Autodesk Inventor part; units mm, degrees
ref_plane "Work Plane2" through (0, 0, 0) normal (-1, 0, 0) x (0, 1, 0)
ref_plane "Work Plane3" through (0, 3.5, 0) normal (0, 1, 0) x (1, 0, 0)
ref_plane "YZ Plane" through (0, 0, 0) normal (1, 0, 0) x (0, 1, 0)
sketch "Sketch3" plane through (0, 0, 0) normal (1, 0, 0) x (0, 1, 0)
  line L0 (0, 0) -> (0, -11) construction
  line L1 (0, 0) -> (7, 0) construction
  line L2 (7, 0) -> (7, -11) construction
  line L3 (0, -11) -> (0, -41.91)
  line L4 (0, -41.91) -> (-1.9706, -41.91) construction
  line L5 (0, -11) -> (7, -11)
  line L6 (7, -11) -> (7, -41.91)
  line L7 (0, -41.91) -> (0, -39.6842) construction
  line L8 (0, -41.91) -> (7, -41.91)
  dimension "d7" = 7
  dimension "d8" = 11
  dimension "d9" = 41.91
revolve "Revolution1" add sketch "Sketch3" angle 360 about axis through (0, 0, 0) along (0, 1, 0)
ref_plane "Work Plane2" through (0, 0, 0) normal (-1, 0, 0) x (0, 1, 0)
sketch "Sketch4" plane through (0, 0, 0) normal (-1, 0, 0) x (0, 1, 0)
  line L0 (0, 0) -> (7, 0)
  line L1 (7, 41.91) -> (7, -41.91)
  line L2 (7, 0) -> (7, 11)
  line L3 (7, 0) -> (8, 0)
  line L4 (8, 0) -> (8, 15)
  line L5 (8, 15) -> (7, 15)
  line L6 (8, 15) -> (8, 41.91)
  line L7 (8, 41.91) -> (7, 41.91)
  line L8 (0, 0) -> (0, 0.75)
  line L9 (0, 11) -> (0, -11)
  line L10 (8, 15) -> (0, 15)
  line L11 (0, 41.91) -> (0, -41.91)
  line L12 (0, 15) -> (-1, 15)
  line L13 (-1, 15) -> (-1, 41.91)
  line L14 (-1, 41.91) -> (0, 41.91)
  dimension "d16" = 11
  dimension "d17" = 1
  dimension "d18" = 15
  dimension "d20" = 0.75
  dimension "d21" = 1
ref_plane "Work Plane3" through (0, 3.5, 0) normal (0, 1, 0) x (1, 0, 0)
revolve "Revolution2" add sketch "Sketch4" angle 360 about axis through (0, 0, 0) along (0, 1, 0) contours L12 L13 L14 L11 | L1 L7 L6 L5
sketch "Sketch5" plane through (0, 8, 0) normal (0, 1, 0) x (1, 0, 0)
  circle A0 centre (0, 0) radius 18.175
  circle A1 centre (0, 0) radius 15
  circle A2 centre (0, 0) radius 41.91
  circle A3 centre (0, 0) radius 35.56
  dimension "d22" = 3.175
  dimension "d23" = 6.35
extrude "Extrusion2" cut sketch "Sketch5" against normal through all contours A3
sketch "Sketch6" plane through (0, 8, 0) normal (0, 1, 0) x (1, 0, 0)
  circle A0 centre (0, 0) radius 18.175
  circle A1 centre (0, 0) radius 35.56
  line L0 (16.0245, 8.5759) -> (30.4464, -18.372)
  line L1 (27.5834, -22.4426) -> (17.7246, -4.0211)
  dimension "d26" = 4.445
extrude "Extrusion3" add sketch "Sketch6" against normal up to surface (9 mm away) contours A0 L0 A1 L1 picked at (22.1844, -5.1361)
pattern_circular "Circular Pattern1" count 3 over 360 about axis through (0, 3.5, 0) along (0, -1, 0) of "Extrusion3"
fillet "Fillet1" radius 6.35 3 edges at (-5.3799, 3.5, -17.3605) (17.7246, 3.5, 4.0211) (-12.3447, 3.5, 13.3394)
fillet "Fillet1" radius 3.175 3 edges at (27.5834, 3.5, 22.4426) (-33.2276, 3.5, 12.6666) (5.6442, 3.5, -35.1092)
fillet "Fillet1" radius 3.175 3 edges at (0.6874, 3.5, -35.5534) (-31.1338, 3.5, 17.1814) (30.4464, 3.5, 18.372)
sketch "Sketch7" plane through (0, 0, 0) normal (-1, 0, 0) x (0, 1, 0)
  line L0 (8, -41.91) -> (8, 41.91)
  line L1 (-1, -41.91) -> (-1, 41.91)
  line L2 (8, -41.91) -> (-1, -41.91)
  arc A0 (6.04, -41.91) -> (8, -35.56) centre (-3.2664, -35.56) ccw
  arc A1 (-1, -35.56) -> (0.96, -41.91) centre (10.2664, -35.56) ccw
  line L3 (0.96, -41.91) -> (6.04, -41.91)
  line L4 (-1, -35.56) -> (8, -35.56)
  line L5 (8, -22.57) -> (-1, -22.57)
  line L6 (8, -24.1718) -> (8, -35.56)
  line L7 (-1, -24.1718) -> (8, -24.1718)
  line L8 (-1, -22.57) -> (-1, -24.1718)
  line L9 (8, -35.56) -> (8, -35.56)
  line L10 (0, 0) -> (11.7377, 0)
  dimension "d36" = 6.35
  dimension "d37" = 5.08
revolve "Revolution3" cut sketch "Sketch7" angle 360 about axis through (0, 0, 0) along (0, 1, 0) contours L2 A0 L0 | A1 L2 L1
fillet "Fillet2" radius 1.5875 4 edges at (41.91, 6.04, 0) (-41.91, 6.04, 0) (-41.91, 0.96, 0) (41.91, 0.96, 0)
sketch "Sketch8" plane through (27.5145, 8, 12.8937) normal (0, 1, 0) x (0.8816766, 0, -0.4718541)
  circle A0 centre (-18.175, 24.3509) radius 19.05
  arc A1 (-27.2625, 8.6109) -> (-12.7058, 7.0183) centre (-18.175, 24.3509) ccw
  dimension "d40" = 38.1
sketch "Sketch9" plane through (27.5145, 8, 12.8937) normal (0, 1, 0) x (0.8816766, 0, -0.4718541)
  circle A0 centre (-18.175, 24.3509) radius 27.1145
  circle A1 centre (-18.175, 24.3509) radius 41.91
  circle A2 centre (-18.175, 24.3509) radius 41.91
  dimension "d41" = 54.229
extrude "Extrusion4" cut sketch "Sketch9" against normal blind 25.4
properties part number "Spinner 1"
Design review of the part built by this model. Coordinates are the model's own, in mm. A direction names the side the tool comes from. Round coordinates to 2 decimals unless told otherwise and drop trailing zeros. Write each loop counter-clockwise with the first axis right and the second up, starting at its lowest first coordinate (ties: lowest second). Pieces come first, ordered by that corner, then holes. Notation, with made-up numbers: M 47,-38.5 L 62,-38.5 A29 cw 62,0.5 Z; hole C -6,46.25 d1. An arc over 180 degrees is marked long. One line per item, written item: value. Start each with the question number.
1. Draft analysis for pull direction Z (two halves, no side actions). For faces 4 (the face through (0.66, -0.507, 14.985)), 5 (the face through (11.295, 3.563, -14.239)), 6 (the face through (-22.39, 3.56, 15.29)), state which applies: pulls with the +Z half, pulls with the -Z half, needs draft (parallel to the pull), parting line crosses it, or undercut.
2. To check wall thickness, follow probe 1 along Z at (x, y) = (3.5, 1); probe 2 along X at (y, z) = (-0.75, 0) (3 decimals); probe 3 along X at (y, z) = (-0.5, -0.5). State the ranges of each line that lie inside material, in increasing order. Write a range as from..to.
3. Take a section at B-B on x = 12. State the section outline as (y, z) points, then the cut area to 3 significant figures.
4. Take a section at A-A on z = -2.5. State the section outline as (x, y) points.
5. Clearance check with flat-ended pins moving along their axes: P1, Ø3, axis at x = -4, z = 10, coming from the +Y side; P2, Ø4, axis at x = 9, z = -2.5, coming from the -Y side; P3, Ø24, axis at x = -1, z = 4.5, coming from the -Y side; P4, Ø1.5, axis at x = -5.5, y = 4.5, coming from the -Z side. State where each tip first meets the part, or that it passes through.
6. For faces 1 (the face through (-10, 0, 5)), 2 (the face through (0.66, 7.493, 14.985)), 3 (the face through (6, -1, 14)), list the 3-axis set-ups (+Z, -Z, +X, -X, +Y, -Y) from which the entire face can be reached by the end or side of a thin tool; tool diameter is ignored.
Computed:
1. face 4: undercut
1. face 5: pulls with the -Z half
1. face 6: pulls with the +Z half
2. probe 1: z = -17.96..-10.43, 10.43..17.83
2. probe 2: x = -18.175..-15, 15..20.614
2. probe 3: x = -18.17..-14.99, 14.99..20.35
3. outline: M -1,-13.65 L 8,-13.65 L 8,-9 L 7,-9 L 7,9 L 8,9 L 8,13.65 L -1,13.65 L -1,9 L 0,9 L 0,-9 L -1,-9 Z
3. area: 210 mm²
4. outline: M -18,-1 L -14.79,-1 L -14.79,0 L -10.71,0 L -10.71,7 L -14.79,7 L -14.79,8 L -18,8 Z; M 10.71,0 L 14.79,0 L 14.79,-1 L 19.28,-1 L 19.28,8 L 14.79,8 L 14.79,7 L 10.71,7 Z
5. P1: stops at y = 7
5. P2: stops at y = 0
5. P3: stops at y = -1
5. P4: stops at z = -26.7
6. face 1: -Y
6. face 2: +Y
6. face 3: +Z, -Z, +X, -X, -Y
